Autodesk Inventor part; units mm, degrees
ref_plane "Work Plane1" through (0, 10, 0) normal (0, 1, 0) x (-1, 0, 0)
sketch "Sketch1" plane through (0, 0, 0) normal (0, 1, 0) x (-1, 0, 0)
  circle A0 centre (0, 0) radius 5
sketch "Sketch2" plane through (0, 10, 0) normal (0, 1, 0) x (-1, 0, 0)
  circle A0 centre (0, 0) radius 3
loft "Loft1" add profiles "Sketch2", "Sketch1"
sketch "Sketch3" plane through (0, 10, 0) normal (0, 1, 0) x (1, 0, 0)
  circle A0 centre (0, 0) radius 3
extrude "Extrusion1" add sketch "Sketch3" along normal blind 60
sketch "Sketch4" plane through (0, 70, 0) normal (0, 1, 0) x (1, 0, 0)
  circle A0 centre (0, 0) radius 1.25
extrude "Extrusion2" cut sketch "Sketch4" against normal blind 80
properties part number "Towers"
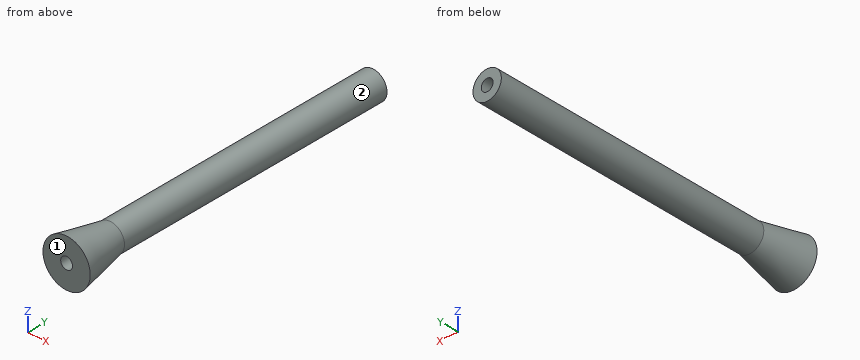
Here's how the part is built. I have some questions about the finished solid (model axes, mm). Face numbers are marked on the shaded views. A direction names the side the tool comes from. Give positions to 0.01 mm unless a question says otherwise; leave off trailing zeros. Loops run counter-clockwise (first coordinate to the right, second up) from the corner with the lowest first, then second, coordinate; pieces in that order, holes last. Notation, with made-up numbers: (65, 68.5) -> (69, 68.5) arc R33 ccw to (69, 103.5) -> close; hole circle Ø3 at (-31.75, -25.5). An arc over 180 degrees is marked (long way). Answer as a JSON object with one key per item and string values. Group by question number.
Item 1: Imagine slicing it at A-A on x = 0. Write out the boundary of the cut face in (y, z), then the cut area to 3 significant figures.
Item 2: Will these pins go through, and if not, where does the flat tip stop? pin 1 (4 mm diameter, centred on y = 13.5, z = 2, fed in from +X); pin 2 (3 mm diameter, centred on x = -3.5, y = 18.5, fed in from +Z); pin 3 (4 mm diameter, centred on y = 16.5, z = -3, fed in from +X).
Item 3: Imagine slicing it at B-B on y = 30. Write out the boundary of the cut face in (x, z), then the cut area to 3 significant figures.
Item 4: On a 3-axis mill with a long thin cutter (end or side, diameter ignored), from which of +Z, -Z, +X, -X, +Y, -Y can I reach the whole of each face in a straight line? I mean the marked faces 1 and 2. Say none if no direction works.
Item 5: I need wall thicknesses on L1, parallel to X at y = 30.5, z = 0; L2, parallel to X at y = 40, z = 0.5. Which ranges of each line are inside material? Lowest first, please.
Answer list:
{
 "1": {"outline": "(0, -5) -> (10, -3) -> (70, -3) -> (70, -1.25) -> (0, -1.25) -> close; (0, 1.25) -> (70, 1.25) -> (70, 3) -> (10, 3) -> (0, 5) -> close", "area": "265 mm2"},
 "2": {"pin 1": "stops at x = 3", "pin 2": "stops at z = 2.24", "pin 3": "stops at x = 2.83"},
 "3": {"outline": "circle Ø6 at (0, 0); hole circle Ø2.5 at (0, 0)", "area": "23.4 mm2"},
 "4": {"face 1": "+Z, -Z, +X, -X, -Y", "face 2": "+Y"},
 "5": {"L1": "x = -3 to -1.25, 1.25 to 3", "L2": "x = -2.96 to -1.15, 1.15 to 2.96"}
}
